Part model, mm, in its own coordinate system. Face numbers are marked on the shaded views. A direction names the side the tool comes from. Coordinates: 2 decimals unless noted, no trailing zeros. Write each loop counter-clockwise with the first axis right and the second up, starting at its lowest first coordinate (ties: lowest second). Pieces come first, ordered by that corner, then holes. Notation, with made-up numbers: (59, -10) - (69, -10) arc R17 cw to (69, 5) - close; hole circle Ø6 at (11.25, 21.25). An arc over 180 degrees is marked (long way). Use a Markdown table: item, result.
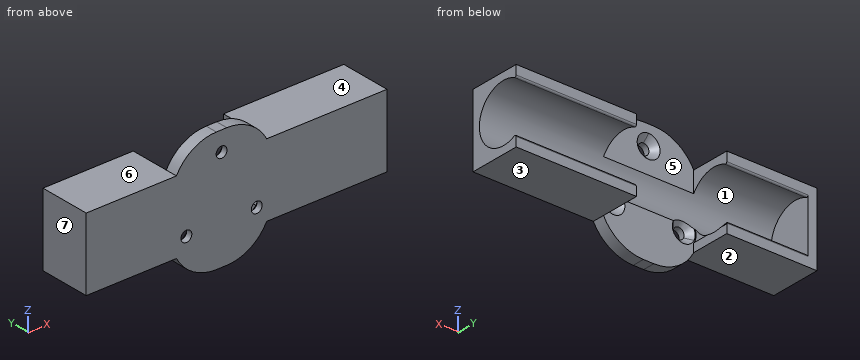
```python
from build123d import *

# Parameters (mm, degrees)
EXTRUDE_2_DEPTH     = 4
SKETCH_7_W          = 100
SKETCH_7_H          = 24
EXTRUDE_3_DEPTH     = 13
SKETCH_8_R          = 9.5
CUT_EXTRUDE_3_DEPTH = 97
SKETCH_9_W          = 30
SKETCH_9_H          = 13
CUT_EXTRUDE_4_DEPTH = 79.822585596
SKETCH_10_R         = 1.8
CUT_EXTRUDE_5_DEPTH = 74.952687578
FILLET_3_R          = 15
FILLET_4_R          = 0.5
CUT_EXTRUDE_9_REACH = 76.76
SKETCH_11_R         = 4.1


with BuildPart() as part:
    # Эскиз6 → Бобышка-Вытянуть2 (new body)
    with BuildSketch(Plane(origin=(0, 0, 0), x_dir=(1, 0, 0), z_dir=(0, 1, 0))):
        Polygon((0, 20), (0, 12), (-30, 12), (-30, -12), (0, -12), (0, -20), (30, -20), (30, -12), (70, -12), (70, 12), (30, 12), (30, 20), align=None)
    extrude(amount=EXTRUDE_2_DEPTH)

    # Эскиз7 → Бобышка-Вытянуть3 (add)
    with BuildSketch(Plane(origin=(0, 4, 0), x_dir=(1, 0, 0), z_dir=(0, 1, 0))):
        with Locations((20, 0)):
            Rectangle(SKETCH_7_W, SKETCH_7_H)
    extrude(amount=EXTRUDE_3_DEPTH)

    # Эскиз8 → Вырез-Вытянуть3 (cut)
    with BuildSketch(Plane(origin=(70, 0, 0), x_dir=(0, 0, -1), z_dir=(1, 0, 0))):
        with Locations((0, 12)):
            Circle(SKETCH_8_R)
    extrude(amount=-CUT_EXTRUDE_3_DEPTH, mode=Mode.SUBTRACT)

    # Эскиз9 → Вырез-Вытянуть4 (cut, through all)
    with BuildSketch(Plane.XY.offset(12)):
        with Locations((15, 10.5)):
            Rectangle(SKETCH_9_W, SKETCH_9_H)
    extrude(amount=-CUT_EXTRUDE_4_DEPTH, mode=Mode.SUBTRACT)

    # Эскиз10 → Вырез-Вытянуть5 (cut, through all)
    with BuildSketch(Plane(origin=(0, 4, 0), x_dir=(1, 0, 0), z_dir=(0, 1, 0))):
        with Locations(Location((15, -13.5, 0), (0, 0, 270))):
            Circle(SKETCH_10_R)
        with Locations(Location((3.308657049, 6.75, 0), (0, 0, 270))):
            Circle(SKETCH_10_R)
        with Locations(Location((26.691342951, 6.75, 0), (0, 0, 270))):
            Circle(SKETCH_10_R)
    extrude(amount=-CUT_EXTRUDE_5_DEPTH, mode=Mode.SUBTRACT)

    # Скругление3
    # the kernel refuses this fillet: 15 mm, written as the material it takes off along each edge
    with BuildSketch(Plane(origin=(30, -33.166247904, -20), x_dir=(-1, 0, 0), z_dir=(0, 1, 0))) as fillet_3_piece_1:
        with BuildLine():
            CenterArc((13.266499161, 15), FILLET_3_R, 207.818139285, 62.181860715)
            Line((0, 8), (-0.265329983, 7.86))
            ThreePointArc((-0.265329983, 7.86), (-0.3, 4), (-0.3, 0))
            Line((-0.3, 0), (0, -0.3))
            Line((0, -0.3), (13.266499161, -0.3))
            Line((13.266499161, -0.3), (13.266499161, 0))
        make_face()
    extrude(amount=70.332495807, mode=Mode.SUBTRACT)
    with BuildSketch(Plane(origin=(0, -33.166247904, -20), x_dir=(0, 0, 1), z_dir=(0, 1, 0))) as fillet_3_piece_2:
        with BuildLine():
            CenterArc((15, 13.266499161), FILLET_3_R, 180, 62.181860715)
            Line((0, 13.266499161), (-0.3, 13.266499161))
            Line((-0.3, 13.266499161), (-0.3, 0))
            Line((-0.3, 0), (0, -0.3))
            ThreePointArc((0, -0.3), (4, -0.3), (7.86, -0.265329983))
            Line((7.86, -0.265329983), (8, 0))
        make_face()
    extrude(amount=70.332495807, mode=Mode.SUBTRACT)
    with BuildSketch(Plane(origin=(30, -33.166247904, 20), x_dir=(-1, 0, 0), z_dir=(0, 1, 0))) as fillet_3_piece_3:
        with BuildLine():
            CenterArc((13.266499161, -15), FILLET_3_R, 90, 62.181860715)
            Line((0, -8), (-0.265329983, -7.86))
            ThreePointArc((-0.265329983, -7.86), (-0.3, -4), (-0.3, 0))
            Line((-0.3, 0), (0, 0.3))
            Line((0, 0.3), (13.266499161, 0.3))
            Line((13.266499161, 0.3), (13.266499161, 0))
        make_face()
    extrude(amount=70.332495807, mode=Mode.SUBTRACT)
    with BuildSketch(Plane(origin=(0, -33.166247904, 20), x_dir=(0, 0, -1), z_dir=(0, 1, 0))) as fillet_3_piece_4:
        with BuildLine():
            CenterArc((15, -13.266499161), FILLET_3_R, 117.818139285, 62.181860715)
            Line((0, -13.266499161), (-0.3, -13.266499161))
            Line((-0.3, -13.266499161), (-0.3, 0))
            Line((-0.3, 0), (0, 0.3))
            ThreePointArc((0, 0.3), (4, 0.3), (7.86, 0.265329983))
            Line((7.86, 0.265329983), (8, 0))
        make_face()
    extrude(amount=70.332495807, mode=Mode.SUBTRACT)

    # Скругление4
    fillet_4_edges = [part.edges().sort_by_distance(p)[0] for p in [
        (50, 17, -8.077747211),
        (-13.5, 17, 8.077747211),
        (50, 17, 8.077747211),
        (-13.5, 17, -8.077747211),
    ]]
    fillet(fillet_4_edges, radius=FILLET_4_R)

    # Вырез-Вытянуть9: up to this face of the body (flat: up to its plane)
    cut_extrude_9_end = Plane(part.part.faces().sort_by_distance((15, 4, 11.690077791))[0])
    # Эскиз11 → Вырез-Вытянуть9 (cut, up to the picked face)
    with BuildSketch(Plane(origin=(0, 17, 0), x_dir=(1, 0, 0), z_dir=(0, 1, 0)), mode=Mode.PRIVATE) as cut_extrude_9_sk1:
        with Locations((15, -13.5)):
            Circle(SKETCH_11_R)
    cut_extrude_9_tool1 = split(extrude(cut_extrude_9_sk1.sketch, amount=-CUT_EXTRUDE_9_REACH, mode=Mode.PRIVATE), bisect_by=cut_extrude_9_end, keep=Keep.BOTH, mode=Mode.PRIVATE)
    # Эскиз11 → Вырез-Вытянуть9 (cut, up to the picked face)
    with BuildSketch(Plane(origin=(0, 17, 0), x_dir=(1, 0, 0), z_dir=(0, 1, 0)), mode=Mode.PRIVATE) as cut_extrude_9_sk2:
        with Locations((3.308657049, 6.75)):
            Circle(SKETCH_11_R)
    cut_extrude_9_tool2 = split(extrude(cut_extrude_9_sk2.sketch, amount=-CUT_EXTRUDE_9_REACH, mode=Mode.PRIVATE), bisect_by=cut_extrude_9_end, keep=Keep.BOTH, mode=Mode.PRIVATE)
    # Эскиз11 → Вырез-Вытянуть9 (cut, up to the picked face)
    with BuildSketch(Plane(origin=(0, 17, 0), x_dir=(1, 0, 0), z_dir=(0, 1, 0)), mode=Mode.PRIVATE) as cut_extrude_9_sk3:
        with Locations((26.691342951, 6.75)):
            Circle(SKETCH_11_R)
    cut_extrude_9_tool3 = split(extrude(cut_extrude_9_sk3.sketch, amount=-CUT_EXTRUDE_9_REACH, mode=Mode.PRIVATE), bisect_by=cut_extrude_9_end, keep=Keep.BOTH, mode=Mode.PRIVATE)
    add(cut_extrude_9_tool1.solids().sort_by(Axis((15, 17, 13.5), (0, -1, 0)))[0], mode=Mode.SUBTRACT)
    add(cut_extrude_9_tool2.solids().sort_by(Axis((3.308657, 17, -6.75), (0, -1, 0)))[0], mode=Mode.SUBTRACT)
    add(cut_extrude_9_tool3.solids().sort_by(Axis((26.691343, 17, -6.75), (0, -1, 0)))[0], mode=Mode.SUBTRACT)

    # Фаска2: read off the stored shape, not the designer's step
    # Фаска2 outline → Фаска2 (revolve, cut)
    with BuildSketch(Plane(origin=(26.691342951, 0, -6.75), x_dir=(1, 0, 0), z_dir=(0, 0, 1))):
        Polygon((1.8, 4.000001023), (1.8, 2), (3.800001023, 4.000001023), align=None)
    revolve(axis=Axis((26.691342951, 0, -6.75), (0, 1, 0)), mode=Mode.SUBTRACT)

    # Фаска1: read off the stored shape, not the designer's step
    # Фаска1: loft between two sections, ruled curve by curve
    chamfer_1_from = [
        Edge.make_three_point_arc((15, 2, 11.7), (13.2, 2, 13.5), (15, 2, 15.3)),
        Edge.make_three_point_arc((15, 2, 15.3), (16.8, 2, 13.5), (15, 2, 11.7)),
    ]
    chamfer_1_to = [
        Edge.make_three_point_arc((15, 4, 9.7), (11.2, 4, 13.5), (15, 4, 17.3)),
        Edge.make_three_point_arc((15, 4, 17.3), (18.8, 4, 13.5), (15, 4, 9.7)),
    ]
    chamfer_1 = Solid(Shell([*[Face.make_surface_from_curves(chamfer_1_from[k], chamfer_1_to[k]) for k in range(2)], Face(Wire(chamfer_1_from)), Face(Wire(chamfer_1_to))]))
    add(chamfer_1, mode=Mode.SUBTRACT)

    # Chamfer 1 2: loft between two sections, ruled curve by curve
    chamfer_1_2_from = [
        Edge.make_three_point_arc((4.935430815, 2, -5.979540971), (4.079116078, 2, -8.376773766), (1.681883283, 2, -7.520459029)),
        Edge.make_three_point_arc((1.681883283, 2, -7.520459029), (2.53819802, 2, -5.123226234), (4.935430815, 2, -5.979540971)),
    ]
    chamfer_1_2_to = [
        Edge.make_three_point_arc((6.742958145, 4.000001023, -5.123474945), (4.935182104, 4.000001023, -10.184301096), (-0.125644047, 4.000001023, -8.376525055)),
        Edge.make_three_point_arc((-0.125644047, 4.000001023, -8.376525055), (1.682131994, 4.000001023, -3.315698904), (6.742958145, 4.000001023, -5.123474945)),
    ]
    chamfer_1_2 = Solid(Shell([*[Face.make_surface_from_curves(chamfer_1_2_from[k], chamfer_1_2_to[k]) for k in range(2)], Face(Wire(chamfer_1_2_from)), Face(Wire(chamfer_1_2_to))]))
    add(chamfer_1_2, mode=Mode.SUBTRACT)


solid = part.part
```
Item 1: Two-plate mould, pull along X, no slides. Class the marked faces 5, 6 and 7: pulls with the +X half, pulls with the -X half, needs draft (parallel to the pull), parting line crosses it, or undercut.
From the geometry:
| item | result |
|---|---|
| face 5 | undercut |
| face 6 | needs draft |
| face 7 | pulls with the -X half |
Item 2: Band-saw the part on A-A, the plane y = 12. Give the cut face in (x, z), then the cut area to 3 significant figures.
From the geometry:
| item | result |
|---|---|
| outline | (-30, -12) - (0, -12) - (0, -9.5) - (-27, -9.5) - (-27, 9.5) - (0, 9.5) - (0, 12) - (-30, 12) - close; (30, -12) - (70, -12) - (70, -9.5) - (30, -9.5) - close; (30, 9.5) - (70, 9.5) - (70, 12) - (30, 12) - close |
| area | 407 mm^2 |
Item 3: Drop flat-ended pins along their axis: P1, Ø10, axis at x = 22, z = 8.5, coming from the -Y side; P2, Ø8.5, axis at x = 49.5, y = 9, coming from the -Z side; P3, Ø7, axis at y = 8.5, z = 1.5, coming from the +X side; P4, Ø3, axis at x = 15, z = 13.5, coming from the +Y side. Give the stop position or say it passes through.
From the geometry:
| item | result |
|---|---|
| P1 | y = 0 |
| P2 | z = -12 |
| P3 | x = -27 |
| P4 | through |
Item 4: Band-saw the part on D-D, the plane x = 8. Give the cut face in (y, z).
From the geometry:
| item | result |
|---|---|
| outline | (0, -19.05) - (4, -19.05) - (4, -5.12) arc R9.5 cw to (4, 5.12) - (4, 19.05) - (0, 19.05) - close |
Item 5: Band-saw the part on C-C, the plane z = 4. Give the cut face in (x, y).
From the geometry:
| item | result |
|---|---|
| outline | (-30, 0) - (70, 0) - (70, 3.38) - (-27, 3.38) - (-27, 17) - (-30, 17) - close |
Item 6: Drill centre lines: probe 1 along X at (y, z) = (1.2, -6.75); probe 2 along X at (y, z) = (3.75, -7); probe 3 along X at (y, z) = (5.25, 7.5). Where is each one in solid material? Low to high.
From the geometry:
| item | result |
|---|---|
| probe 1 | -30 to 1.51, 5.11 to 24.89, 28.49 to 70 |
| probe 2 | -30 to -0.23, 6.85 to 23.15, 30.23 to 70 |
| probe 3 | -30 to 0, 30 to 70 |
Item 7: Band-saw the part on B-B, the plane x = -21. Give the cut face in (y, z) (3 decimals).
From the geometry:
| item | result |
|---|---|
| outline | (0, -12) - (17, -12) - (17, -8.93) arc R0.5 ccw to (16.275, -8.484) arc R9.5 cw (long way) to (16.275, 8.484) arc R0.5 ccw to (17, 8.93) - (17, 12) - (0, 12) - close |
Item 8: Which spindle directions (+Z, -Z, +X, -X, +Y, -Y) get a long thin tool onto all of the face, cutting with end or side? Do the marked faces 1, 2, 3 and 4. Say none if no direction does.
From the geometry:
| item | result |
|---|---|
| face 1 | +X |
| face 2 | -Z, -X, +Y, -Y |
| face 3 | -Z, +X, +Y, -Y |
| face 4 | +Z, +X, +Y, -Y |
